Verification items for the finished model (mm, model axes). A direction names the side the tool comes from. Round coordinates to 2 decimals unless told otherwise and drop trailing zeros. Order: outer loops, then holes, each group sorted by start corner. A loop starts at its lowest first (then second) coordinate and runs counter-clockwise, first axis right, second up. Notation, with made-up numbers: (14, -10) -> (57, -10) arc R10 ccw to (57, -3) -> close; hole circle Ø10 at (54, 83). An arc over 180 degrees is marked (long way). Return JSON: item names as keys, results as strings. Group by question number.
1) Tool access check on faces 1 (the cylindrical face through (3.226, -17.67, 5.059)), 2 (the cylindrical face through (-1.08, 5.42, -4.88)), 3 (the cylindrical face through (6.466, -5.923, -2.681)). Record the directions out of +Z, -Z, +X, -X, +Y, -Y that give a thin tool (end or side, any length) a straight path to the whole face; none if there is none.
2) Depth check by flat-ended pin: pin 1 (3 mm diameter, centred on y = -9.5, z = -2.5, fed in from -X); pin 2 (1 mm diameter, centred on x = 4.5, z = -5.5, fed in from +Y); pin 3 (5 mm diameter, centred on x = 4, y = 7, fed in from -Z); pin 4 (3.5 mm diameter, centred on x = 0, y = -18, fed in from +Z). Enter the tip coordinate at first touch or a pass-through.
3) Section check A-A on x = 0. Enter the section's corners in (y, z), plus the area to 3 significant figures.
4) Section check D-D on y = -4. Enter the section's corners in (x, z), plus the area to 3 significant figures.
5) Scan lines: L1, parallel to Y at x = 0, z = 4; L2, parallel to Y at x = -2.25, z = 2; L3, parallel to X at y = -18, z = -1.75. Record each from-to range of solid material in increasing order.
6) Section check C-C on y = -18. Enter the section's corners in (x, z).
7) Section check B-B on y = 10. Enter the section's corners in (x, z), plus the area to 3 significant figures.
```python
from build123d import *

# Parameters (mm, degrees)
F0_R          = 7
F0_R_2        = 6
F1_DEPTH      = 12
F0_R_3        = 5
F2_DEPTH      = 24
F3_DEPTH      = 24
F3_DEPTH_BACK = 12
F4_SIZE       = 1
F5_SIZE       = 0.5
F6_R          = 3
F7_DEPTH      = 25
F7_DEPTH_BACK = 25


with BuildPart() as f1:
    # F0 (on Front) → F1 (new body)
    with BuildSketch(Plane.XZ):
        Circle(F0_R)
        Circle(F0_R_2, mode=Mode.SUBTRACT)
    extrude(amount=F1_DEPTH)

    # F0 (on Front) → F2 (join)
    with BuildSketch(Plane.XZ):
        Circle(F0_R_2)
        Circle(F0_R_3, mode=Mode.SUBTRACT)
    extrude(amount=F2_DEPTH)

    # F0 (on Front) → F3 (join, two sides)
    with BuildSketch(Plane.XZ) as f3_sk:
        Circle(F0_R_3)
    extrude(amount=F3_DEPTH)
    extrude(f3_sk.sketch, amount=-F3_DEPTH_BACK)

    # F4
    f4_edges = [f1.edges().sort_by_distance(p)[0] for p in [
        (-5, 12, 0),
    ]]
    chamfer(f4_edges, length=F4_SIZE)

    # F5
    f5_edges = [f1.edges().sort_by_distance(p)[0] for p in [
        (-6, -24, 0),
        (-7, -12, 0),
        (7, -6, 0),
        (-7, 0, 0),
    ]]
    chamfer(f5_edges, length=F5_SIZE)

    # F6 (on Top) → F7 (cut, two sides)
    with BuildSketch(Plane.XY) as f7_sk:
        with Locations((0, -18)):
            Circle(F6_R)
    extrude(amount=-F7_DEPTH, mode=Mode.SUBTRACT)
    extrude(f7_sk.sketch, amount=F7_DEPTH_BACK, mode=Mode.SUBTRACT)


solid = f1.part
```
Check result:
{
 "1": {"face 1": "-Y", "face 2": "+Y", "face 3": "+Y, -Y"},
 "2": {"pin 1": "x = -6.93", "pin 2": "y = -0.11", "pin 3": "z = -4.77", "pin 4": "through"},
 "3": {"outline": "(-24, -5.5) -> (-23.5, -6) -> (-21, -6) -> (-21, 6) -> (-23.5, 6) -> (-24, 5.5) -> close; (-15, -6) -> (-12, -6) -> (-12, -6.5) -> (-11.5, -7) -> (-0.5, -7) -> (0, -6.5) -> (0, -5) -> (11, -5) -> (12, -4) -> (12, 4) -> (11, 5) -> (0, 5) -> (0, 6.5) -> (-0.5, 7) -> (-11.5, 7) -> (-12, 6.5) -> (-12, 6) -> (-15, 6) -> close", "area": "358 mm^2"},
 "4": {"outline": "circle Ø14 at (0, 0)", "area": "154 mm^2"},
 "5": {"L1": "-24 to -21, -15 to 12", "L2": "-24 to -19.98, -16.02 to 12", "L3": "-5.74 to -3, 3 to 5.74"},
 "6": {"outline": "(-3, -5.2) -> (-3, 5.2) arc R6 ccw to start; (3, -5.2) arc R6 ccw to (3, 5.2) -> close"},
 "7": {"outline": "circle Ø10 at (0, 0)", "area": "78.5 mm^2"}
}
